For this review, take the finished solid that the model builds, in its own axes (mm). Face numbers are marked on the shaded views. A direction names the side the tool comes from. Round coordinates to 2 decimals unless told otherwise and drop trailing zeros. Write each loop counter-clockwise with the first axis right and the second up, starting at its lowest first coordinate (ties: lowest second). Pieces come first, ordered by that corner, then holes. Notation, with made-up numbers: (3.25, -4.75) -> (39.25, -4.75) arc R29 ccw to (39.25, 20.25) -> close; hole circle Ø1 at (51, 40.25). An arc over 180 degrees is marked (long way). Answer as CSV lines item,"result". Start each with the question number.
Item 1: Wall thickness on probe 1 along X at (y, z) = (5, -31); probe 2 along Y at (x, z) = (-18, -48); probe 3 along Z at (x, y) = (-4.5, 57.5): over which ranges is each line inside the solid? List them lowest first. Write a range as from..to.
Item 2: Mouldability with a two-part tool opening along X and no side actions: class the marked faces 3, 4, 5 and 6 as +X half, -X half, draft (parallel to the pull), parting line (faces both ways), or undercut.
Item 3: Take a section at B-B on y = 3.64. Give the boundary of the cut face in (x, z), then the cut area to 3 significant figures.
Item 4: Take a section at D-D on y = 35. Give the boundary of the cut face in (x, z).
Item 5: Machinability: for the marked faces 1 and 2, which of the approach directions +Z, -Z, +X, -X, +Y, -Y give a long, thin tool a straight path to every point of the face, cutting with its end or side? Answer none if there is none.
Item 6: For pin 1 Ø2.5 at (x, z) = (-30.9, -68.4) entering from -Y; pin 2 Ø3 at (x, y) = (30.9, 3.64) entering from +Z; pin 3 Ø8 at (x, y) = (6, 33) entering from -Z; pin 4 Ø5 at (x, z) = (-29, -10.5) entering from +Y (3 decimals), all flat-tipped, find the tip position at first contact; note any pin that passes through.
Item 7: Take a section at A-A on x = 30.9. Give the boundary of the cut face in (y, z).
Item 8: Take a section at C-C on z = -18. Give the boundary of the cut face in (x, y), then the cut area to 3 significant figures.
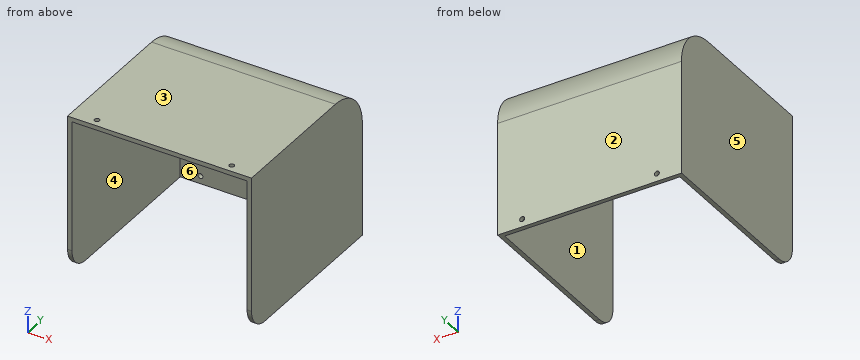
```python
from build123d import *

# Parameters (mm, degrees)
BOSS_EXTRUDE1_DEPTH = 42.2
SKETCH2_R           = 1.15
CUT_EXTRUDE1_DEPTH  = 70
FILLET1_R           = 20
BOSS_EXTRUDE2_DEPTH = 2
FILLET2_R           = 10
SKETCH4_R           = 1.15
CUT_EXTRUDE2_DEPTH  = 10


with BuildPart() as part:
    # Sketch1 → Boss-Extrude1 (new body, symmetric)
    with BuildSketch(Plane(origin=(0, 0, 0), x_dir=(0, 0, -1), z_dir=(1, 0, 0))):
        Polygon((0, 0), (0, 82.2), (72, 82.2), (72, 80.2), (2, 80.2), (2, 0), align=None)
    extrude(amount=BOSS_EXTRUDE1_DEPTH, both=True)

    # Sketch2 → Cut-Extrude1 (cut)
    with BuildSketch(Plane.XY):
        with Locations((-30.9, 3.64)):
            Circle(SKETCH2_R)
        with Locations((30.9, 3.64)):
            Circle(SKETCH2_R)
    extrude(amount=-CUT_EXTRUDE1_DEPTH, mode=Mode.SUBTRACT)

    # Fillet1
    fillet1_edges = [part.edges().sort_by_distance(p)[0] for p in [
        (0, 82.2, 0),
        (0, 80.2, -2),
    ]]
    fillet(fillet1_edges, radius=FILLET1_R)

    # Sketch3 → Boss-Extrude2 (add)
    with BuildSketch(Plane.ZY.offset(42.2)):
        with BuildLine():
            Line((-72, 80.2), (-72, 0))
            Line((-72, 0), (-2, 0))
            Line((-2, 0), (-2, 60.2))
            ThreePointArc((-2, 60.2), (-7.857864376, 74.342135624), (-22, 80.2))
            Line((-22, 80.2), (-72, 80.2))
        make_face()
    boss_extrude2 = extrude(amount=-BOSS_EXTRUDE2_DEPTH)

    # Mirror1: Boss-Extrude2 across plane
    add(boss_extrude2.mirror(Plane(origin=(0, 0, 0), x_dir=(0, 0, 1), z_dir=(1, 0, 0))))

    # Fillet2
    fillet2_edges = [part.edges().sort_by_distance(p)[0] for p in [
        (-41.2, 0, -72),
        (41.2, 0, -72),
    ]]
    fillet(fillet2_edges, radius=FILLET2_R)

    # Sketch4 → Cut-Extrude2 (cut)
    with BuildSketch(Plane(origin=(0, 82.2, 0), x_dir=(1, 0, 0), z_dir=(0, 1, 0))):
        with Locations((-30.9, 68.401968)):
            Circle(SKETCH4_R)
        with Locations((30.9, 68.401968)):
            Circle(SKETCH4_R)
    extrude(amount=-CUT_EXTRUDE2_DEPTH, mode=Mode.SUBTRACT)


solid = part.part
```
Output values:
1,probe 1,"x = -42.2..-40.2, 40.2..42.2"
1,probe 2,"y = 80.2..82.2"
1,probe 3,"z = -2..0"
2,face 3,"draft"
2,face 4,"undercut"
2,face 5,"-X half"
2,face 6,"undercut"
3,outline,"(-42.2, -69.72) -> (-40.2, -69.72) -> (-40.2, -2) -> (-32.05, -2) -> (-32.05, 0) -> (-42.2, 0) -> close; (-29.75, -2) -> (29.75, -2) -> (29.75, 0) -> (-29.75, 0) -> close; (32.05, -2) -> (40.2, -2) -> (40.2, -69.72) -> (42.2, -69.72) -> (42.2, 0) -> (32.05, 0) -> close"
3,area,"430 mm^2"
4,outline,"(-42.2, -72) -> (-40.2, -72) -> (-40.2, -2) -> (40.2, -2) -> (40.2, -72) -> (42.2, -72) -> (42.2, 0) -> (-42.2, 0) -> close"
5,face 1,"-Z, -Y"
5,face 2,"+Z, -Z, +X, -X, +Y"
6,pin 1,"stops at y = 80.2"
6,pin 2,"stops at z = 0"
6,pin 3,"stops at z = -2"
6,pin 4,"stops at y = 80.935"
7,outline,"(0, -2) -> (2.49, -2) -> (2.49, 0) -> (0, 0) -> close; (4.79, -2) -> (60.2, -2) arc R20 cw to (80.2, -22) -> (80.2, -67.25) -> (82.2, -67.25) -> (82.2, -20) arc R20 ccw to (62.2, 0) -> (4.79, 0) -> close; (80.2, -72) -> (82.2, -72) -> (82.2, -69.55) -> (80.2, -69.55) -> close"
8,outline,"(-42.2, 0) -> (-40.2, 0) -> (-40.2, 79.8) -> (40.2, 79.8) -> (40.2, 0) -> (42.2, 0) -> (42.2, 82.1) -> (-42.2, 82.1) -> close"
8,area,"514 mm^2"
